Study the drawing (mm; zero at the part's minimum x, y, z) and answer. Coordinates: 2 decimals unless noted, no trailing zeros. Order: outer loops, then holes, each group sorted by start corner. A loop starts at its lowest first (then second) coordinate and runs counter-clockwise, first axis right, second up. Notation, with made-up numbers: (-24, 61.5) -> (-16, 61.5) arc R13 ccw to (-16, 65.5) -> close; hole circle Ø7 at (86, -7.5). An arc over 180 degrees is marked (long way). Answer in a Markdown table with one row per item. Add a question column.
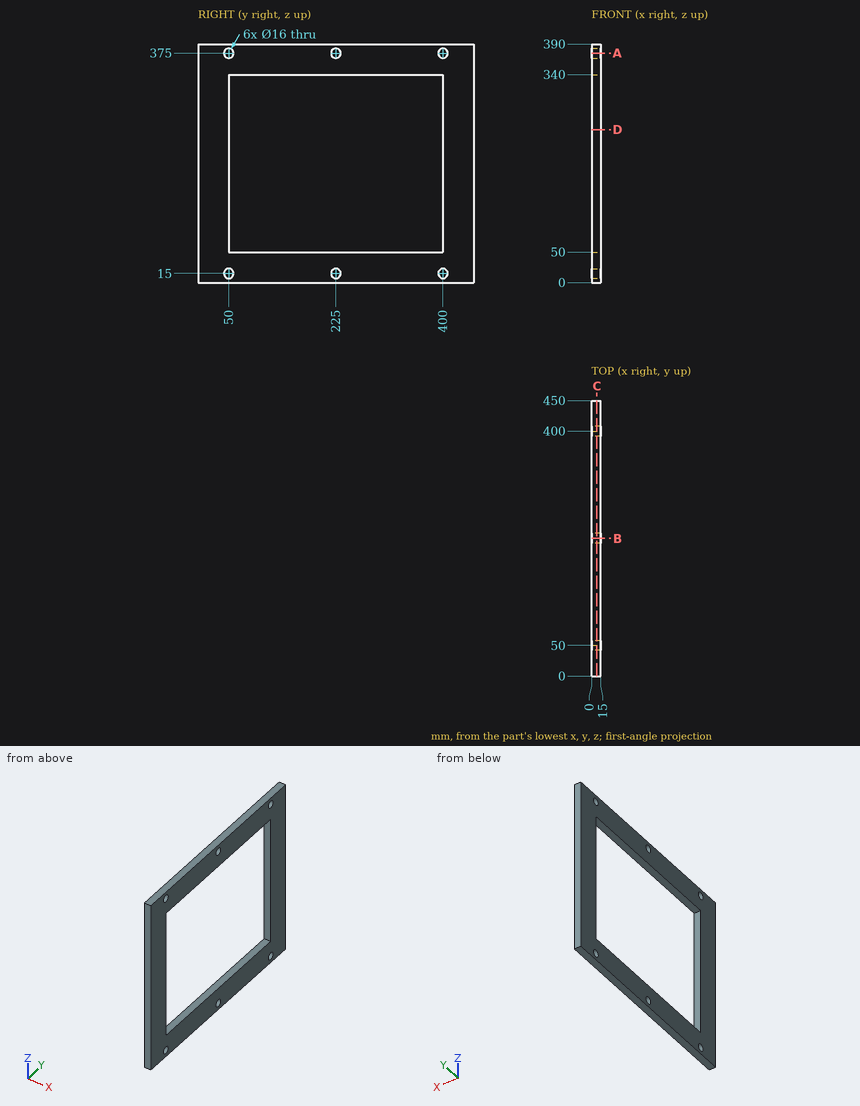
Q1. A cutting plane is placed at D-D (z = 250). Determine the outline of the cut face in (x, y), then the cut area to 3 significant figures.
Q2. A cutting plane is placed at B-B (y = 225). Determine the outline of the cut face in (x, z), then the cut area to 3 significant figures.
Q3. Straight lines are drawn through the part: line 1 (Y direction, x = 9, z = 375); line 2 (Z direction, x = 5.25, y = 278); line 3 (Y direction, x = 8.25, z = 99.5). For each, find the intervals that lie inside material, in ascending order.
Q4. A cutting plane is placed at A-A (z = 375). Determine the outline of the cut face in (x, y), then the cut area to 3 significant figures.
Q5. A cutting plane is placed at C-C (x = 8.75). Determine the outline of the cut face in (y, z), then the cut area to 3 significant figures.
Returned:
| question | item | result |
|---|---|---|
| 1 | outline | (0, 0) -> (15, 0) -> (15, 50) -> (0, 50) -> close; (0, 400) -> (15, 400) -> (15, 450) -> (0, 450) -> close |
| 1 | area | 1,500 mm² |
| 2 | outline | (0, 0) -> (15, 0) -> (15, 7) -> (0, 7) -> close; (0, 23) -> (15, 23) -> (15, 50) -> (0, 50) -> close; (0, 340) -> (15, 340) -> (15, 367) -> (0, 367) -> close; (0, 383) -> (15, 383) -> (15, 390) -> (0, 390) -> close |
| 2 | area | 1,020 mm² |
| 3 | line 1 | y = 0 to 42, 58 to 217, 233 to 392, 408 to 450 |
| 3 | line 2 | z = 0 to 50, 340 to 390 |
| 3 | line 3 | y = 0 to 50, 400 to 450 |
| 4 | outline | (0, 0) -> (15, 0) -> (15, 42) -> (0, 42) -> close; (0, 58) -> (15, 58) -> (15, 217) -> (0, 217) -> close; (0, 233) -> (15, 233) -> (15, 392) -> (0, 392) -> close; (0, 408) -> (15, 408) -> (15, 450) -> (0, 450) -> close |
| 4 | area | 6,030 mm² |
| 5 | outline | (0, 0) -> (450, 0) -> (450, 390) -> (0, 390) -> close; hole circle Ø16 at (50, 15); hole circle Ø16 at (50, 375); hole (50, 50) -> (400, 50) -> (400, 340) -> (50, 340) -> close; hole circle Ø16 at (225, 15); hole circle Ø16 at (225, 375); hole circle Ø16 at (400, 15); hole circle Ø16 at (400, 375) |
| 5 | area | 72,800 mm² |
